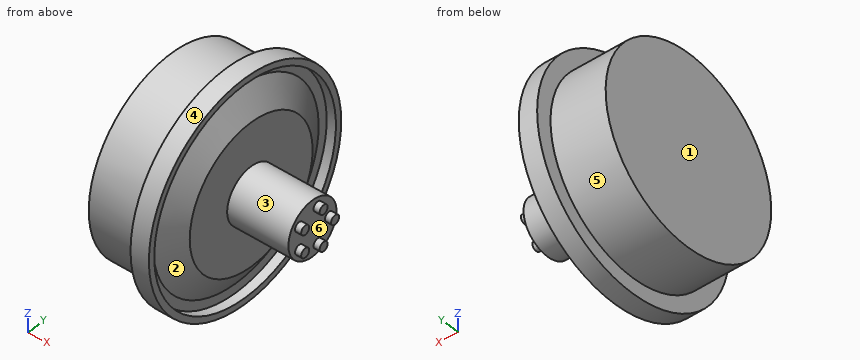
from build123d import *

# Parameters (mm, degrees)
SKETCH4_R           = 0.75
BOSS_EXTRUDE2_DEPTH = 1


with BuildPart() as part:
    # Sketch1 → Revolve1 (revolve)
    with BuildSketch(Plane(origin=(0, 0, 0), x_dir=(1, 0, 0), z_dir=(0, 1, 0))):
        Polygon((-7.620406457, 0), (-7.620406457, 15.5), (1.379593543, 15.5), (1.379593543, 18), (3.379593543, 18), (4.379593543, 18), (4.379593543, 17), (3.379593543, 17), (2.879593543, 17), (2.879593543, 15.5), (5.379593543, 11.5), (5.379593543, 4.5), (15.379593543, 4.5), (15.379593543, 3.7), (15.379593543, 0), (14.579593543, 0), (5.379593543, 0), align=None)
    revolve(axis=Axis((-25, 0, 0), (1, 0, 0)))

    # Sketch4 → Boss-Extrude2 (add)
    with BuildSketch(Plane(origin=(15.379593543, 0, 0), x_dir=(0, 0, -1), z_dir=(1, 0, 0))):
        with Locations((0, 3.093773222)):
            Circle(SKETCH4_R)
        with Locations((2.942353182, 0.956028502)):
            Circle(SKETCH4_R)
        with Locations((1.818474274, -2.502915113)):
            Circle(SKETCH4_R)
        with Locations((-1.818474274, -2.502915113)):
            Circle(SKETCH4_R)
        with Locations((-2.942353182, 0.956028502)):
            Circle(SKETCH4_R)
    extrude(amount=BOSS_EXTRUDE2_DEPTH)


solid = part.part
Can you work these out from the model? Positions are in its coordinate system, mm. Face numbers are marked on the shaded views. A direction names the side the tool comes from. Give positions to 0.01 mm unless a question says otherwise; leave off trailing zeros. Loops run counter-clockwise (first coordinate to the right, second up) from the corner with the lowest first, then second, coordinate; pieces in that order, holes last. Notation, with made-up numbers: (89, -17) -> (142, -17) arc R19 ccw to (142, 11) -> close; hole circle Ø2 at (75, -15.5). An arc over 180 degrees is marked (long way). Write item = value, one per line.
1) I need wall thicknesses on L1, parallel to Y at x = 3.6, z = 0; L2, parallel to Z at x = 3.75, y = -1; L3, parallel to X at y = -13, z = -10.5. Which ranges of each line are inside material? Lowest first, please. Write a range as from..to.
Check result:
L1 = -18..-17, -14.35..14.35, 17..18
L2 = -17.97..-16.97, -14.07..14.07, 16.97..17.97
L3 = 1.38..2.88
2) For the marked faces 4, 5 and 6, which set-ups out of +Z, -Z, +X, -X, +Y, -Y let a thin tool reach every point of the face, with its end or its side?
Check result:
face_4 = +X, -X
face_5 = -X
face_6 = +X
3) Suppose I cut it at B-B on x = 13. Write out the boundary of the cut face in (y, z), then the cut area to 3 significant figures.
Check result:
outline = circle Ø9 at (0, 0)
area = 63.6 mm2
4) Thinking about a two-plate mould opening in Y: for the marked faces 1, 2 and 3, which applies, released by +Y, released by -Y, zero draft, split by the parting line, or undercut?
Check result:
face_1 = zero draft
face_2 = undercut
face_3 = split by the parting line
5) Will these pins go through, and if not, where does the flat tip stop? pin 1 (3 mm diameter, centred on x = 12, z = 1.5, fed in from -Y); pin 2 (5 mm diameter, centred on x = 13, y = -2, fed in from -Z); pin 3 (3 mm diameter, centred on x = 5, y = -12, fed in from -Z).
Check result:
pin_1 = -4.5
pin_2 = -4.5
pin_3 = -14.52
6) Suppose I cut it at A-A on z = 0. Write out the boundary of the cut face in (x, y), then the cut area to 3 significant figures.
Check result:
outline = (-7.62, -15.5) -> (1.38, -15.5) -> (1.38, -18) -> (4.38, -18) -> (4.38, -17) -> (2.88, -17) -> (2.88, -15.5) -> (5.38, -11.5) -> (5.38, -4.5) -> (15.38, -4.5) -> (15.38, 2.34) -> (16.38, 2.34) -> (16.38, 3.84) -> (15.38, 3.84) -> (15.38, 4.5) -> (5.38, 4.5) -> (5.38, 11.5) -> (2.88, 15.5) -> (2.88, 17) -> (4.38, 17) -> (4.38, 18) -> (1.38, 18) -> (1.38, 15.5) -> (-7.62, 15.5) -> close
area = 495 mm2
